Source: CAD feature listing. Evaluate the final solid. Frame: model axes, mm. Coordinates: 2 decimals unless noted, no trailing zeros. Order: outer loops, then holes, each group sorted by start corner. A loop starts at its lowest first (then second) coordinate and runs counter-clockwise, first axis right, second up.
```python
from build123d import *

# Parameters (mm, degrees)
SKETCH2_W           = 51.27
SKETCH2_H           = 26.65
BOSS_EXTRUDE2_DEPTH = 5
SKETCH3_W           = 45.27
SKETCH3_H           = 20.65
CUT_EXTRUDE1_DEPTH  = 6
SKETCH4_W           = 3.75
SKETCH4_H           = 3.75
BOSS_EXTRUDE3_DEPTH = 5
SKETCH5_R           = 1.12
CUT_EXTRUDE2_DEPTH  = 6
SKETCH6_W           = 15
SKETCH6_H           = 108
BOSS_EXTRUDE4_DEPTH = 5
SKETCH7_W           = 10
SKETCH7_H           = 20
BOSS_EXTRUDE5_DEPTH = 5
SKETCH8_R           = 1.75
CUT_EXTRUDE3_DEPTH  = 6
SKETCH9_W           = 15
SKETCH9_H           = 0.2
CUT_EXTRUDE4_DEPTH  = 6


with BuildPart() as part:
    # Sketch2 → Boss-Extrude2 (new body)
    with BuildSketch(Plane(origin=(0, 0, 0), x_dir=(1, 0, 0), z_dir=(0, 1, 0))):
        with Locations((22.635, 10.325)):
            Rectangle(SKETCH2_W, SKETCH2_H)
    extrude(amount=BOSS_EXTRUDE2_DEPTH)

    # Sketch3 → Cut-Extrude1 (cut, through all)
    with BuildSketch(Plane(origin=(0, 5, 0), x_dir=(1, 0, 0), z_dir=(0, 1, 0))):
        with Locations((22.635, 10.325)):
            Rectangle(SKETCH3_W, SKETCH3_H)
    extrude(amount=-CUT_EXTRUDE1_DEPTH, mode=Mode.SUBTRACT)

    # Sketch4 → Boss-Extrude3 (add)
    with BuildSketch(Plane(origin=(0, 5, 0), x_dir=(1, 0, 0), z_dir=(0, 1, 0))):
        with Locations((1.875, 18.775)):
            Rectangle(SKETCH4_W, SKETCH4_H)
        with Locations((1.875, 1.875)):
            Rectangle(SKETCH4_W, SKETCH4_H)
        with Locations((43.395, 1.875)):
            Rectangle(SKETCH4_W, SKETCH4_H)
        with Locations((43.395, 18.775)):
            Rectangle(SKETCH4_W, SKETCH4_H)
    extrude(amount=-BOSS_EXTRUDE3_DEPTH)

    # Sketch5 → Cut-Extrude2 (cut, through all)
    with BuildSketch(Plane(origin=(0, 5, 0), x_dir=(1, 0, 0), z_dir=(0, 1, 0))):
        with Locations((1.385, 18.975)):
            Circle(SKETCH5_R)
        with Locations((43.885, 18.975)):
            Circle(SKETCH5_R)
        with Locations((43.885, 1.675)):
            Circle(SKETCH5_R)
        with Locations((1.385, 1.675)):
            Circle(SKETCH5_R)
    extrude(amount=-CUT_EXTRUDE2_DEPTH, mode=Mode.SUBTRACT)

    # Sketch6 → Boss-Extrude4 (add)
    with BuildSketch(Plane(origin=(0, 5, 0), x_dir=(1, 0, 0), z_dir=(0, 1, 0))):
        with Locations((22.635, -57)):
            Rectangle(SKETCH6_W, SKETCH6_H)
    extrude(amount=-BOSS_EXTRUDE4_DEPTH)

    # Sketch7 → Boss-Extrude5 (add)
    with BuildSketch(Plane(origin=(0, 5, 0), x_dir=(1, 0, 0), z_dir=(0, 1, 0))):
        with Locations((35.135, -111)):
            Rectangle(SKETCH7_W, SKETCH7_H)
        with Locations((10.135, -111)):
            Rectangle(SKETCH7_W, SKETCH7_H)
    extrude(amount=-BOSS_EXTRUDE5_DEPTH)

    # Sketch8 → Cut-Extrude3 (cut, through all)
    with BuildSketch(Plane(origin=(0, 5, 0), x_dir=(1, 0, 0), z_dir=(0, 1, 0))):
        with Locations((10.135, -116)):
            Circle(SKETCH8_R)
        with Locations((35.135, -116)):
            Circle(SKETCH8_R)
    extrude(amount=-CUT_EXTRUDE3_DEPTH, mode=Mode.SUBTRACT)

    # Sketch9 → Cut-Extrude4 (cut, through all)
    with BuildSketch(Plane(origin=(0, 5, 0), x_dir=(1, 0, 0), z_dir=(0, 1, 0))):
        with Locations((22.635, -110.9)):
            Rectangle(SKETCH9_W, SKETCH9_H)
    extrude(amount=-CUT_EXTRUDE4_DEPTH, mode=Mode.SUBTRACT)


solid = part.part
```
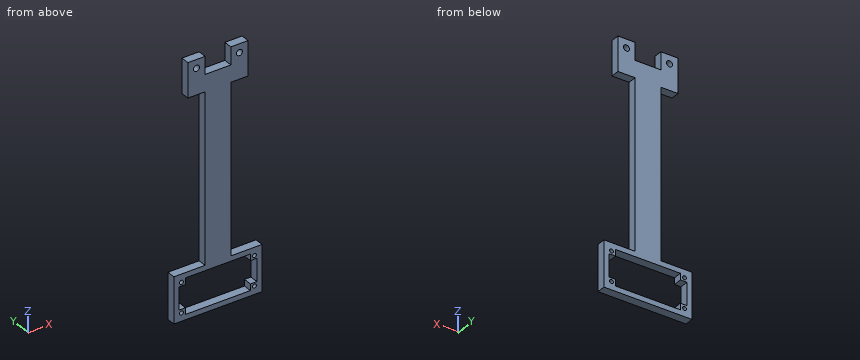
1. Section query B-B on x = 18.5. Return loops of the section in (y, z), plus the area to 3 significant figures.
Findings:
outline: (0, -23.65) - (5, -23.65) - (5, -20.65) - (0, -20.65) - close; (0, 0) - (5, 0) - (5, 110.8) - (0, 110.8) - close
area: 569 mm2
2. Section query C-C on x = 31.5. Return loops of the section in (y, z).
Findings:
outline: (0, -23.65) - (5, -23.65) - (5, -20.65) - (0, -20.65) - close; (0, 0) - (5, 0) - (5, 3) - (0, 3) - close; (0, 101) - (5, 101) - (5, 121) - (0, 121) - close
3. Section query D-D on y = 0.85. Count the separate pieces of the cut face and the enclosed holes in it, plus the area to 3 significant figures.
Findings:
separate pieces: 1
enclosed holes: 7
area: 2,470 mm2
4. Section query A-A on z = 116. Return loops of the section in (x, y) (3 decimals).
Findings:
outline: (5.135, 0) - (8.385, 0) - (8.385, 5) - (5.135, 5) - close; (11.885, 0) - (15.135, 0) - (15.135, 5) - (11.885, 5) - close; (30.135, 0) - (33.385, 0) - (33.385, 5) - (30.135, 5) - close; (36.885, 0) - (40.135, 0) - (40.135, 5) - (36.885, 5) - close
5. Ray query, line 1 (X direction, y = 1.1, z = 116) (3 decimals); line 2 (Z direction, x = 38, y = 0.8); line 3 (Z direction, x = 17, y = 1.45). Return the intervals inside material, ascending.
Findings:
line 1: x = 5.135 to 8.385, 11.885 to 15.135, 30.135 to 33.385, 36.885 to 40.135
line 2: z = -23.65 to -20.65, 0 to 3, 101 to 121
line 3: z = -23.65 to -20.65, 0 to 110.8
6. Pin query (flat end, axial travel): P1, Ø1.5, axis at y = 3, z = 70.5, coming from the -X side (3 decimals); P2, Ø2.5, axis at y = 3.5, z = 108, coming from the -X side (3 decimals); P3, Ø3, axis at y = 1, z = 20.5, coming from the +X side (3 decimals). Return the tip coordinate at first contact, or that it passes through.
Findings:
P1: stops at x = 15.135
P2: stops at x = 5.135
P3: stops at x = 30.135
